Autodesk Inventor part; units mm, degrees
ref_plane "YZ Plane" through (0, 0, 0) normal (1, 0, 0) x (0, 1, 0)
ref_plane "XZ Plane" through (0, 0, 0) normal (0, 1, 0) x (-1, 0, 0)
ref_plane "XY Plane" through (0, 0, 0) normal (0, 0, 1) x (1, 0, 0)
sketch "Sketch1" plane through (0, 0, 0) normal (0, 1, 0) x (-1, 0, 0)
  line L0 (0, 0) -> (10, 0)
  line L1 (10, 0) -> (10, -20)
  line L2 (10, -20) -> (0, -20)
  line L3 (0, -20) -> (0, 0)
  dimension "d0" = 20
  dimension "d1" = 10
extrude "Extrusion1" add sketch "Sketch1" along normal blind 6
sketch "Sketch2" plane through (0, 6, 0) normal (0, 1, 0) x (1, 0, 0)
  circle A0 centre (-6, 5.25) radius 1.1
  circle A1 centre (-6, 14.75) radius 1.1
  line L0 (-10, 20) -> (-10, 0)
  line L1 (0, 20) -> (-10, 20)
  point P0 (0, 0)
  dimension "d4" = 2.2
  dimension "d5" = 2.2
  dimension "d6" = 9.5
  dimension "d7" = 4
  dimension "d8" = 4
  dimension "d9" = 5.25
extrude "Extrusion2" cut sketch "Sketch2" against normal blind 6
sketch "Sketch3" plane through (0, 6, 0) normal (0, 1, 0) x (1, 0, 0)
  line L0 (-1.1092, 1.7066) -> (4.0185, 19.8124)
  line L1 (4.0185, 19.8124) -> (5.4927, 19.3949)
  line L2 (-10, 0) -> (0, 0)
  line L3 (5.4927, 19.3949) -> (0, 0)
  line L4 (-1.1092, 1.7066) -> (0, 0)
extrude "Extrusion3" add sketch "Sketch3" against normal blind 6
fillet "Fillet1" radius 1 13 edges at (0, 6, -12.8116) (0, 3, -20) (-5, 6, -20) (-5, 0, -20) (-5, 6, 0) (-10, 6, -10) (-10, 3, 0) (-10, 0, -10) (-10, 3, -20) (-5, 0, 0) (0, 3, 0) (0, 0, -12.8116) (4.0185, 3, -19.8124)
properties part number "Endstop"
Geometry: final body of the model. Coordinates: model frame, mm. A direction names the side the tool comes from. Coordinates: 2 decimals unless noted, no trailing zeros. Order: outer loops, then holes, each group sorted by start corner. A loop starts at its lowest first (then second) coordinate and runs counter-clockwise, first axis right, second up. Notation, with made-up numbers: (28.5, 3) - (58.5, 3) arc R19 ccw to (58.5, 23) - close; hole circle Ø11 at (22.25, -4). An arc over 180 degrees is marked (long way). Return JSON: item names as keys, results as strings. Group by question number.
1. Set-up query: faces 1 (the face through (-4.944, 5.699, -19.715)), 2 (the face through (-4.944, 0.285, -19.699)), 3 (the face through (-0.285, 5.699, -12.306)). Return all of +Z, -Z, +X, -X, +Y, -Y with unobstructed straight access to the full face (end or side cutting, diameter ignored); none if empty.
2. Cut plane B-B (z = -5.25). Output: boundary loops of the cut face in (x, y), plus the area to 3 significant figures.
3. Pin query (flat end, axial travel): pin 1 (2 mm diameter, centred on y = 3.5, z = -8, fed in from +X); pin 2 (1.3 mm diameter, centred on x = -6, z = -14.75, fed in from +Y); pin 3 (2 mm diameter, centred on y = 2, z = -10, fed in from +X). Return the tip coordinate at first contact, or that it passes through.
4. Pull-direction query (Z, two-part tool) for faces 4 (the face through (-5.41, 3.04, -6.18)), 5 (the face through (2.886, 3.042, -10.192)), 6 (the face through (-3, 0, -10)); classes: pulls with the +Z half, pulls with the -Z half, needs draft (parallel to the pull), parting line crosses it, or undercut.
5. Cut plane C-C (y = 3.4). Output: boundary loops of the cut face in (x, z), plus the area to 3 significant figures.
6. Cut plane A-A (x = -6). Output: boundary loops of the cut face in (y, z).
7. Cut plane D-D (z = -14.75). Output: boundary loops of the cut face in (x, y), plus the area to 3 significant figures.
8. Material intervals for line 1 along Z through (x, y) = (-6, 3.6); line 2 along X through (y, z) = (1.95, -14.75); line 3 along X through (y, z) = (1.65, -15.5), sorted ascending. Write a range as [from, to].
Resolved:
{
 "1": {"face 1": "-Z, -X, +Y", "face 2": "-Z, -X, -Y", "face 3": "-Z, +Y"},
 "2": {"outline": "(-10, 1) arc R1 ccw to (-9, 0) - (-7.1, 0) - (-7.1, 6) - (-9, 6) arc R1 ccw to (-10, 5) - close; (-4.9, 0) - (-1, 0) arc R1 ccw to (-0.11, 0.55) - (-0.11, 0) - (1.49, 0) - (1.49, 6) - (-0.11, 6) - (-0.11, 5.45) arc R1 ccw to (-1, 6) - (-4.9, 6) - close", "area": "55.0 mm²"},
 "3": {"pin 1": "stops at x = 2.55", "pin 2": "passes through", "pin 3": "stops at x = 3.12"},
 "4": {"face 4": "undercut", "face 5": "pulls with the +Z half", "face 6": "needs draft"},
 "5": {"outline": "(-10, -19) arc R1 ccw to (-9, -20) - (-1, -20) arc R1 ccw to (0, -19) - (0, -5.62) - (3.75, -18.85) arc R1 ccw to (4.98, -19.54) - (5.49, -19.39) - (0.21, -0.73) arc R1 ccw to (-0.76, 0) - (-9, 0) arc R1 ccw to (-10, -1) - close; hole circle Ø2.2 at (-6, -14.75); hole circle Ø2.2 at (-6, -5.25)", "area": "218 mm²"},
 "6": {"outline": "(0, -19) arc R1 ccw to (1, -20) - (5, -20) arc R1 ccw to (6, -19) - (6, -15.85) - (0, -15.85) - close; (0, -13.65) - (6, -13.65) - (6, -6.35) - (0, -6.35) - close; (0, -4.15) - (6, -4.15) - (6, -1) arc R1 ccw to (5, 0) - (1, 0) arc R1 ccw to (0, -1) - close"},
 "7": {"outline": "(-10, 1) arc R1 ccw to (-9, 0) - (-7.1, 0) - (-7.1, 6) - (-9, 6) arc R1 ccw to (-10, 5) - close; (-4.9, 0) - (-1, 0) arc R1 ccw to (0, 1) - (0, 5) arc R1 ccw to (-1, 6) - (-4.9, 6) - close; (2.58, 0) - (4.18, 0) - (4.18, 6) - (2.58, 6) - close", "area": "55.5 mm²"},
 "8": {"line 1": "z = [-20, -15.85], [-13.65, -6.35], [-4.15, 0]", "line 2": "x = [-10, -7.1], [-4.9, 0], [2.58, 4.18]", "line 3": "x = [-10, -6.8], [-5.2, 0], [2.8, 4.39]"}
}
